CAD build for the part. Positions are in the model's coordinates, mm. A direction names the side the tool comes from. Give positions to 0.01 mm unless a question says otherwise; leave off trailing zeros. Write each loop counter-clockwise with the first axis right and the second up, starting at its lowest first coordinate (ties: lowest second). Pieces come first, ordered by that corner, then holes. Notation, with made-up numbers: (39.25, -37) - (50.25, -37) arc R11 cw to (50.25, -17) - close; hole circle Ø4 at (74.25, 46.5). An arc over 180 degrees is marked (long way). Answer as a JSON object with one key per item and string values.
from build123d import *

# Parameters (mm, degrees)
BOSS_EXTRUDE1_DEPTH                            = 30
SKETCH2_W                                      = 80
SKETCH2_H                                      = 26
BOSS_EXTRUDE2_DEPTH                            = 8
CBORE_FOR_M3_HEX_SOCKET_HEAD_CAP_SCR_2_COUNT   = 2
CBORE_FOR_M3_HEX_SOCKET_HEAD_CAP_SCR_2_PITCH   = 45
SKETCH5_W                                      = 12
SKETCH5_H                                      = 26
CUT_EXTRUDE1_DEPTH                             = 8
FILLET1_R                                      = 4
CBORE_FOR_M3_HEX_SOCKET_HEAD_CAP_SCR_3_COUNT   = 2
CBORE_FOR_M3_HEX_SOCKET_HEAD_CAP_SCR_3_PITCH   = 68.951359668
CBORE_FOR_M3_HEX_SOCKET_HEAD_CAP_SCR_4_COUNT   = 2
CBORE_FOR_M3_HEX_SOCKET_HEAD_CAP_SCR_4_PITCH   = 67.3
CBORE_FOR_M3_HEX_SOCKET_HEAD_CAP_SCR_5_COUNT   = 2
CBORE_FOR_M3_HEX_SOCKET_HEAD_CAP_SCR_5_PITCH   = 15
CBORE_START                                    = -10
CBORE_SLOT_FOR_M6_HEX_SOCKET_HEAD_CAP_SC_DEPTH = 4
CBORE_START_2                                  = -14
CBORE_SLOT_FOR_M6_HEX_SOCKET_HEAD_CA_3_DEPTH   = 4
CHAMFER1_SIZE                                  = 0.4


# Read off the part's stored shape, not the designer's step: CBORE SLOT for M6 Hex Socket Head Cap Screw2
with BuildPart() as part:
    # Sketch1 → Boss-Extrude1 (new body)
    with BuildSketch(Plane(origin=(0, 0, 0), x_dir=(1, 0, 0), z_dir=(0, 1, 0))):
        Polygon((-40, 14), (-40, 0), (-27.3, 0), (-27.3, 6), (27.3, 6), (27.3, 0), (40, 0), (40, 14), align=None)
    extrude(amount=BOSS_EXTRUDE1_DEPTH)

    # Sketch2 → Boss-Extrude2 (add)
    with BuildSketch(Plane.XZ):
        with Locations((0, -27)):
            Rectangle(SKETCH2_W, SKETCH2_H)
    extrude(amount=-BOSS_EXTRUDE2_DEPTH)

    # Sketch4 → CBORE for M3 Hex Socket Head Cap Screw1 (revolve, cut)
    with BuildSketch(Plane(origin=(-22.5, 0, -26.5), x_dir=(0, 0, -1), z_dir=(1, 0, 0))):
        Polygon((0, 0), (0, 21.021463052), (1.7, 20), (1.7, 3.4), (3.25, 3.4), (3.25, 0.025), (3.275, 0), align=None)
    cbore_for_m3_hex_socket_head_cap_screw1 = revolve(axis=Axis((-22.5, -6.35, -26.5), (0, 1, 0)), mode=Mode.SUBTRACT)

    # CBORE for M3 Hex Socket Head Cap Scr 2: CBORE for M3 Hex Socket Head Cap Screw1 ×2
    with Locations(*[(i * CBORE_FOR_M3_HEX_SOCKET_HEAD_CAP_SCR_2_PITCH, 0, 0) for i in range(1, CBORE_FOR_M3_HEX_SOCKET_HEAD_CAP_SCR_2_COUNT)]):
        add(cbore_for_m3_hex_socket_head_cap_screw1, mode=Mode.SUBTRACT)

    # Sketch5 → Cut-Extrude1 (cut)
    with BuildSketch(Plane.XZ):
        with Locations((-34, -27)):
            Rectangle(SKETCH5_W, SKETCH5_H)
        with Locations((34, -27)):
            Rectangle(SKETCH5_W, SKETCH5_H)
    extrude(amount=-CUT_EXTRUDE1_DEPTH, mode=Mode.SUBTRACT)

    # Fillet1
    fillet1_edges = [part.edges().sort_by_distance(p)[0] for p in [
        (28, 4, -40),
        (-28, 4, -40),
    ]]
    fillet(fillet1_edges, radius=FILLET1_R)

    # Sketch7 → CBORE for M3 Hex Socket Head Cap Screw2 (revolve, cut)
    with BuildSketch(Plane(origin=(33.65, 22.5, -14), x_dir=(0, 1, 0), z_dir=(1, 0, 0))):
        Polygon((0, 0), (0, 21.021463052), (1.7, 20), (1.7, 4.4), (3.25, 4.4), (3.25, 0.025), (3.275, 0), align=None)
    cbore_for_m3_hex_socket_head_cap_screw2 = revolve(axis=Axis((33.65, 22.5, -20.35), (0, 0, 1)), mode=Mode.SUBTRACT)

    # CBORE for M3 Hex Socket Head Cap Scr 3: CBORE for M3 Hex Socket Head Cap Screw2 ×2
    with Locations(*[Vector(-0.9760503683250792, -0.2175446586162881, 0) * (i * CBORE_FOR_M3_HEX_SOCKET_HEAD_CAP_SCR_3_PITCH) for i in range(1, CBORE_FOR_M3_HEX_SOCKET_HEAD_CAP_SCR_3_COUNT)]):
        add(cbore_for_m3_hex_socket_head_cap_screw2, mode=Mode.SUBTRACT)

    # CBORE for M3 Hex Socket Head Cap Scr 4: CBORE for M3 Hex Socket Head Cap Screw2 ×2
    with Locations(*[(-i * CBORE_FOR_M3_HEX_SOCKET_HEAD_CAP_SCR_4_PITCH, 0, 0) for i in range(1, CBORE_FOR_M3_HEX_SOCKET_HEAD_CAP_SCR_4_COUNT)]):
        add(cbore_for_m3_hex_socket_head_cap_screw2, mode=Mode.SUBTRACT)

    # CBORE for M3 Hex Socket Head Cap Scr 5: CBORE for M3 Hex Socket Head Cap Screw2 ×2
    with Locations(*[(0, -i * CBORE_FOR_M3_HEX_SOCKET_HEAD_CAP_SCR_5_PITCH, 0) for i in range(1, CBORE_FOR_M3_HEX_SOCKET_HEAD_CAP_SCR_5_COUNT)]):
        add(cbore_for_m3_hex_socket_head_cap_screw2, mode=Mode.SUBTRACT)

    # CBORE SLOT for M6 Hex Socket Head Ca 2 → CBORE SLOT for M6 Hex Socket Head Cap Screw2 (cut)
    with BuildSketch(Plane.XY.offset(CBORE_START)):
        with BuildLine():
            Line((7, 16.5), (7, 21.5))
            ThreePointArc((7, 21.5), (0, 28.5), (-7, 21.5))
            Line((-7, 21.5), (-7, 16.5))
            ThreePointArc((-7, 16.5), (0, 9.5), (7, 16.5))
        make_face()
    extrude(amount=CBORE_SLOT_FOR_M6_HEX_SOCKET_HEAD_CAP_SC_DEPTH, mode=Mode.SUBTRACT)

    # CBORE SLOT for M6 Hex Socket Head Ca 3 o → CBORE SLOT for M6 Hex Socket Head Ca 3 (cut)
    with BuildSketch(Plane.XY.offset(CBORE_START_2)):
        with BuildLine():
            Line((3.5, 16.5), (3.5, 21.5))
            ThreePointArc((3.5, 21.5), (0, 25), (-3.5, 21.5))
            Line((-3.5, 21.5), (-3.5, 16.5))
            ThreePointArc((-3.5, 16.5), (0, 13), (3.5, 16.5))
        make_face()
    extrude(amount=CBORE_SLOT_FOR_M6_HEX_SOCKET_HEAD_CA_3_DEPTH, mode=Mode.SUBTRACT)

    # Chamfer1
    chamfer1_edges = [part.edges().sort_by_distance(p)[0] for p in [
        (33.65, 20.8, 0),
        (40, 0, -7),
        (33.65, 5.8, 0),
        (33.65, 0, 0),
        (-33.65, 30, 0),
        (27.3, 0, -3),
        (-33.65, 20.8, 0),
        (0, 0, -6),
        (-27.3, 0, -3),
        (-33.65, 5.8, 0),
        (-33.65, 0, 0),
        (3.5, 19, -14),
        (0, 13, -14),
        (0, 25, -14),
        (-3.5, 19, -14),
        (-3.5, 19, -10),
        (7, 19, -6),
        (0, 28.5, -6),
        (0, 9.5, -6),
        (0, 25, -10),
        (0, 13, -10),
        (3.5, 19, -10),
        (-7, 19, -6),
        (-27.3, 30, -3),
        (-40, 15, -14),
        (40, 15, -14),
        (40, 15, 0),
        (27.3, 15, 0),
        (-27.3, 15, 0),
        (-40, 15, 0),
        (0, 30, -6),
        (27.3, 30, -3),
        (33.65, 30, 0),
        (40, 30, -7),
        (0, 30, -14),
        (-22.5, 8, -24.8),
        (22.5, 8, -24.8),
        (-40, 30, -7),
        (-40, 0, -7),
        (34, 0, -14),
        (-34, 0, -14),
        (-28, 0, -25),
        (-28, 8, -25),
        (28, 0, -25),
        (0, 0, -40),
        (26.828427125, 0, -38.828427125),
        (-26.828427125, 0, -38.828427125),
        (0, 8, -40),
        (28, 8, -25),
        (26.828427125, 8, -38.828427125),
        (-26.828427125, 8, -38.828427125),
    ]]
    chamfer(chamfer1_edges, length=CHAMFER1_SIZE)


solid = part.part
Item 1: Probe line 1 (X direction, y = 6.7, z = -26.5); line 2 (Y direction, x = 33.65, z = -11.65); line 3 (X direction, y = 7.5, z = -7). List the from-to ranges inside material, lowest first. Write a range as from..to.
Entries:
{"line 1": "-28..-24.2, -20.8..20.8, 24.2..28", "line 2": "0..4.25, 10.75..19.25, 25.75..30", "line 3": "-40..-35.35, -31.95..31.95, 35.35..40"}
Item 2: Cut at B-B (x = 22.5). Give the cut face in (y, z) (3 decimals).
Entries:
{"outline": "(0, -39.6) - (0.4, -40) - (7.6, -40) - (8, -39.6) - (8, -28.6) - (7.6, -28.2) - (3.4, -28.2) - (3.4, -29.75) - (0.025, -29.75) - (0, -29.775) - close; (0, -23.225) - (0.025, -23.25) - (3.4, -23.25) - (3.4, -24.8) - (7.6, -24.8) - (8, -24.4) - (8, -14) - (29.6, -14) - (30, -13.6) - (30, -6.4) - (29.6, -6) - (0.4, -6) - (0, -6.4) - close"}
Item 3: Flat gauge pins, fed straight in: P1, Ø1.5, axis at x = -26, y = 23, coming from the +Z side; P2, Ø5.5, axis at x = 33.65, y = 7.5, coming from the +Z side; P3, Ø7, axis at x = -33, y = 8.5, coming from the -Z side; P4, Ø8, axis at y = 2.5, z = -29, coming from the -X side. Where does each tip first touch, or does it go through?
Entries:
{"P1": "z = -6", "P2": "z = 0", "P3": "z = -14", "P4": "x = -28"}
Item 4: Cut at A-A (z = -26.5). State how many separate pieces and enclosed holes the cut face has, and give its area (3 significant figures).
Entries:
{"separate pieces": "3", "enclosed holes": "0", "area": "372 mm2"}
Item 5: Which spindle directions (+Z, -Z, +X, -X, +Y, -Y) get a long thin tool onto all of the face, cutting with end or side? Do faces 5 (the cylindrical face through (23.745, 1.689, -29.502)), 6 (the conical face through (0.08, 25.11, -13.71)), 7 (the cylindrical face through (-0.15, 9.5, -8.23)). Say none if no direction does.
Entries:
{"face 5": "-Y", "face 6": "-Z", "face 7": "+Z"}
Item 6: Cut at C-C (z = -12.5). Give the cut face in (x, y), and give its area (3 significant figures).
Entries:
{"outline": "(-40, 0.4) - (-39.6, 0) - (39.6, 0) - (40, 0.4) - (40, 29.6) - (39.6, 30) - (-39.6, 30) - (-40, 29.6) - close; hole circle Ø6.5 at (-33.65, 7.5); hole circle Ø6.5 at (-33.65, 22.5); hole (-3.5, 16.5) arc R3.5 ccw to (3.5, 16.5) - (3.5, 21.5) arc R3.5 ccw to (-3.5, 21.5) - close; hole circle Ø6.5 at (33.65, 7.5); hole circle Ø6.5 at (33.65, 22.5)", "area": "2,190 mm2"}
Item 7: Cut at D-D (x = 0). Give the cut face in (y, z).
Entries:
{"outline": "(0, -39.6) - (0.4, -40) - (7.6, -40) - (8, -39.6) - (8, -14) - (12.6, -14) - (13, -13.6) - (13, -10.4) - (12.6, -10) - (9.5, -10) - (9.5, -6.4) - (9.1, -6) - (0.4, -6) - (0, -6.4) - close; (25, -13.6) - (25.4, -14) - (29.6, -14) - (30, -13.6) - (30, -6.4) - (29.6, -6) - (28.9, -6) - (28.5, -6.4) - (28.5, -10) - (25.4, -10) - (25, -10.4) - close"}
Item 8: Mould opens along Z. For faces 1 (the flat face through (-1, 0, -20)), 2 (the cylindrical face through (-23.01, 5.47, -28.12)), 3 (the conical face through (-0.08, 12.89, -10.29)), 4 (the conical face through (-26.593, 7.892, -38.651)) say: +Z half, -Z half, draft (parallel to the pull), parting line (faces both ways), or undercut.
Entries:
{"face 1": "draft", "face 2": "undercut", "face 3": "+Z half", "face 4": "-Z half"}
